Could you check a few things on this model? Use its own coordinates, in mm. A direction names the side the tool comes from. Give positions to 0.01 mm unless a question says otherwise; leave off trailing zeros. Loops run counter-clockwise (first coordinate to the right, second up) from the corner with the lowest first, then second, coordinate; pieces in that order, holes last. Notation, with made-up numbers: (75, 7) - (88, 7) arc R21 cw to (88, 16) - close; hole circle Ø6 at (-21.75, -7.5). An arc over 180 degrees is marked (long way). Write each question's results on one line, items separated by ' | '. Start each with the question number.
1) On a 3-axis mill with a long thin cutter (end or side, diameter ignored), from which of +Z, -Z, +X, -X, +Y, -Y can I reach the whole of each face in a straight line? I mean faces 1 (the face through (-21.141, -5.883, 20.854)), 2 (the face through (-14, 12, 12.5)), 3 (the face through (-22.33, 11.72, 20.52)). Say none if no direction works.
2) I want a section at B-B, the plane y = 0. Write out the boundary of the cut face in (x, z), and give its area (3 significant figures).
3) I want a section at D-D, the plane z = 9.75. Write out the boundary of the cut face in (x, y), and give its area (3 significant figures).
4) I want a section at A-A, the plane x = 2.25. Write out the boundary of the cut face in (y, z), and give its area (3 significant figures).
5) I want a section at C-C, the plane x = -7.75. Write out the boundary of the cut face in (y, z).
6) If we mould it in two halves opening along Y, with no side actions, what happens to faces 4 (the face through (-15, 14.1, 10)), 5 (the face through (-21, -6, 12.5)), 6 (the face through (-9.83, 12, 9))? For each: +Y half, -Y half, draft (parallel to the pull), parting line (faces both ways), or undercut.
7) I'm going to push flat-ended pins straight in: pin 1 (4 mm diameter, centred on x = -21.5, y = 11, fed in from -Z); pin 2 (3.5 mm diameter, centred on y = -11.5, z = 7.5, fed in from +X); pin 3 (1.4 mm diameter, centred on x = -14, y = 11.5, fed in from -Z). Where does each tip first touch, or does it pass through?
8) If I drill on probe 1 along X at (y, z) = (-11.5, 20.7) (3 decimals); probe 2 along Y at (x, z) = (-13.75, 10.75); probe 3 along Y at (x, z) = (-21.33, 19.85) (3 decimals), over which ranges is the centre line in solid material (lowest first)? Write a range as [from, to].
Autodesk Inventor part; units mm, degrees
ref_plane "Work Plane4" through (-37.83, -24.85, 0) normal (0, 0, -1) x (0, 1, 0)
ref_plane "YZ Plane" through (0, 0, 0) normal (1, 0, 0) x (0, 1, 0)
ref_plane "XZ Plane" through (0, 0, 0) normal (0, 1, 0) x (-1, 0, 0)
ref_plane "Work Plane3" through (-9.83, 0, 22) normal (0, 0, -1) x (0, -1, 0)
sketch "Sketch2" plane through (-9.83, 0, 22) normal (0, 0, -1) x (0, -1, 0)
  line L0 (14, 11.5) -> (14, -11.5) construction
  arc A0 (14, 11.5) -> (11.5, 14) centre (11.5, 11.5) ccw construction
  line L1 (-11.5, 14) -> (11.5, 14) construction
  arc A1 (-11.5, 14) -> (-14, 11.5) centre (-11.5, 11.5) ccw construction
  line L2 (-14, -11.5) -> (-14, 11.5) construction
  arc A2 (-14, -11.5) -> (-11.5, -14) centre (-11.5, -11.5) ccw construction
  line L3 (11.5, -14) -> (-11.5, -14) construction
  arc A3 (11.5, -14) -> (14, -11.5) centre (11.5, -11.5) ccw construction
  circle A4 centre (0, 0) radius 11 construction
  circle A5 centre (-11.5, 11.5) radius 1.025 construction
  circle A6 centre (11.5, 11.5) radius 1.025 construction
  circle A7 centre (11.5, -11.5) radius 1.025 construction
  circle A8 centre (-11.5, -11.5) radius 1.025 construction
  line L4 (14.1, -11.5) -> (14.1, 11.5)
  arc A9 (14.1, 11.5) -> (11.5, 14.1) centre (11.5, 11.5) ccw
  line L5 (11.5, 14.1) -> (-11.5, 14.1)
  arc A10 (-11.5, 14.1) -> (-14.1, 11.5) centre (-11.5, 11.5) ccw
  line L6 (-14.1, 11.5) -> (-14.1, -11.5)
  arc A11 (-14.1, -11.5) -> (-11.5, -14.1) centre (-11.5, -11.5) ccw
  line L7 (-11.5, -14.1) -> (11.5, -14.1)
  arc A12 (11.5, -14.1) -> (14.1, -11.5) centre (11.5, -11.5) ccw
  circle A13 centre (0, 0) radius 12.75
  circle A14 centre (-11.5, -11.5) radius 1.025
  circle A15 centre (11.5, -11.5) radius 1.025
  circle A16 centre (11.5, 11.5) radius 1.025
  circle A17 centre (-11.5, 11.5) radius 1.025
  point P0 (0, -9.83)
  dimension "d3" = 0.1
  dimension "d4" = 25.5
  dimension "d5" = 0
  dimension "d6" = 0
  dimension "d7" = 0
  dimension "d8" = 0
extrude "Extrusion2" add sketch "Sketch2" along normal blind 3
sketch "Sketch3" plane through (-9.83, 0, 19) normal (0, 0, -1) x (-1, 0, 0)
  circle A0 centre (0, 0) radius 12.75
  circle A1 centre (11.5, 11.5) radius 1.025
  circle A2 centre (11.5, -11.5) radius 1.025
  circle A3 centre (-11.5, -11.5) radius 1.025
  circle A4 centre (-11.5, 11.5) radius 1.025
  line L0 (-11.5, -14.1) -> (11.5, -14.1)
  arc A5 (11.5, -14.1) -> (14.1, -11.5) centre (11.5, -11.5) ccw
  line L1 (14.1, -11.5) -> (14.1, 11.5)
  arc A6 (14.1, 11.5) -> (11.5, 14.1) centre (11.5, 11.5) ccw
  line L2 (11.5, 14.1) -> (-11.5, 14.1)
  arc A7 (-11.5, 14.1) -> (-14.1, 11.5) centre (-11.5, 11.5) ccw
  line L3 (-14.1, 11.5) -> (-14.1, -11.5)
  arc A8 (-14.1, -11.5) -> (-11.5, -14.1) centre (-11.5, -11.5) ccw
  line L4 (-11.5, -14.1) -> (11.5, -14.1)
  line L5 (0, -14.1) -> (0, -12.75)
  line L6 (0, 12.75) -> (0, 14.1)
  line L7 (11.5, 14.1) -> (-11.5, 14.1)
  circle A9 centre (0, 0) radius 10
  line L8 (0, -10) -> (0, -12.75)
  line L9 (0, 10) -> (0, 12.75)
  point P0 (-9.83, 0)
  dimension "d11" = 20
ref_plane "Work Plane4" through (-37.83, -24.85, 0) normal (0, 0, -1) x (0, 1, 0)
extrude "Extrusion3" add sketch "Sketch3" along normal blind 21.5 contours A0 L8 A9 L9 | A0 L6 L2 A6 L1 A5 L0 L5 picked at (11.7268, -0.9457)
sketch "Sketch4" plane through (-9.83, -14.1, -2.5) normal (0, 0, -1) x (-1, 0, 0)
  circle A0 centre (4.2632, 2.351) radius 1.4
  circle A1 centre (11.5541, 7.5847) radius 1.4
  arc A2 (0, 4.1) -> (0, 24.1) centre (0, 14.1) ccw
  line L0 (10, 14.1) -> (14.0989, 14.1)
  circle A3 centre (4.2632, 25.849) radius 1.4
  circle A4 centre (11.5541, 20.6153) radius 1.4
  point P0 (-9.83, 14.1)
  dimension "d16" = 2.8
  dimension "d17" = 2.8
extrude "Extrusion4" cut sketch "Sketch4" against normal blind 15
sketch "Sketch5" plane through (-9.83, -14.1, -2.5) normal (0, 0, -1) x (-1, 0, 0)
  circle A0 centre (11.5, 2.6) radius 1.025
  circle A1 centre (11.5, 25.6) radius 1.025
  circle A2 centre (11.5, 2.6) radius 2.6
  circle A3 centre (11.5, 25.6) radius 2.6
  point P0 (-9.83, 14.1)
  point P1 (14.1, 2.6)
  dimension "d11" = 20
extrude "Extrusion5" cut sketch "Sketch5" against normal up to surface (21.5 mm away) contours A0 | A1 | A2 | A3
sketch "Sketch6" plane through (-9.83, 0, 19) normal (0, 0, -1) x (-1, 0, 0)
  circle A0 centre (-11.5, 11.5) radius 1.025
  circle A1 centre (-11.5, -11.5) radius 1.025
  line L0 (0, -14.1) -> (0, -12.75)
  arc A2 (0, 12.75) -> (0, -12.75) centre (0, 0) ccw
  line L1 (0, 12.75) -> (0, 14.1)
  line L2 (0, 14.1) -> (-11.5, 14.1)
  arc A3 (-11.5, 14.1) -> (-14.1, 11.5) centre (-11.5, 11.5) ccw
  line L3 (-14.1, 11.5) -> (-14.1, -11.5)
  arc A4 (-14.1, -11.5) -> (-11.5, -14.1) centre (-11.5, -11.5) ccw
  line L4 (-11.5, -14.1) -> (0, -14.1)
  point P0 (-9.83, 0)
extrude "Extrusion6" cut sketch "Sketch6" against normal blind 1
properties part number "30_Cube_Z_Focus_MGN_NEMA_Motoradapter_NEMA11_v3"
Answers:
1) face 1: +Z | face 2: -Z | face 3: +Z, -Z
2) outline: (-23.93, -2.5) - (-19.83, -2.5) - (-19.83, 19) - (-22.58, 19) - (-22.58, 22) - (-23.93, 22) - close; (2.92, 20) - (4.27, 20) - (4.27, 22) - (2.92, 22) - close | area: 94.9 mm2
3) outline: (-23.93, -11.5) arc R2.6 cw (long way) to (-21.33, -14.1) - (-9.83, -14.1) - (-9.83, -10) arc R10 cw to (-9.83, 10) - (-9.83, 14.1) - (-21.33, 14.1) arc R2.6 cw (long way) to (-23.93, 11.5) - close; hole circle Ø2.8 at (-21.38, -6.52); hole circle Ø2.8 at (-21.38, 6.52); hole circle Ø2.8 at (-14.09, -11.75); hole circle Ø2.8 at (-14.09, 11.75) | area: 171 mm2
4) outline: (-14.03, 20) - (-12.35, 20) - (-12.35, 22) - (-14.03, 22) - close; (-10.65, 20) - (-4.08, 20) - (-4.08, 22) - (-10.65, 22) - close; (4.08, 20) - (10.65, 20) - (10.65, 22) - (4.08, 22) - close; (12.35, 20) - (14.03, 20) - (14.03, 22) - (12.35, 22) - close | area: 33.1 mm2
5) outline: (-14.1, 20) - (-12.58, 20) - (-12.58, 22) - (-14.1, 22) - close; (12.58, 20) - (14.1, 20) - (14.1, 22) - (12.58, 22) - close
6) face 4: +Y half | face 5: undercut | face 6: draft
7) pin 1: stops at z = 19 | pin 2: stops at x = -9.83 | pin 3: stops at z = 12.5
8) probe 1: x = [-23.93, -22.355], [-20.305, -15.336], [-4.324, 0.645], [2.695, 4.27] | probe 2: y = [-14.1, -13.11], [-10.39, -9.2], [9.2, 10.39], [13.11, 14.1] | probe 3: y = [-14.1, -12.525], [-10.475, -5.506], [5.506, 10.475], [12.525, 14.1]
